Read the model definition and answer for the solid it produces. Units are mm, in the model's axes. Face numbers are marked on the shaded views. A direction names the side the tool comes from. Round coordinates to 2 decimals unless told otherwise and drop trailing zeros. Write each loop counter-clockwise with the first axis right and the second up, starting at its lowest first coordinate (ties: lowest second). Pieces come first, ordered by that corner, then holes. Notation, with made-up numbers: (-36.5, 47) -> (-20.5, 47) arc R8 cw to (-20.5, 53) -> close; hole circle Ø7 at (59.5, -37). An arc over 180 degrees is marked (long way). Return JSON: item names as keys, results as strings. Group by question number.
(1) The mould has two halves that part along Y. Classify the marked faces 1, 2 and 3: released by +Y, released by -Y, zero draft, split by the parting line, or undercut.
(2) A cutting plane is placed at B-B on y = 57. Give the vertices of the cut face in (x, z), then the cut area to 3 significant figures.
(3) A cutting plane is placed at D-D on x = 68.5. Give the vertices of the cut face in (y, z), then the cut area to 3 significant figures.
(4) A cutting plane is placed at A-A on x = 25. Give the vertices of the cut face in (y, z).
(5) A cutting plane is placed at C-C on z = -23. Give the vertices of the cut face in (x, y).
(6) Given pin 1 (6 mm diameter, centred on x = 26.5, y = 55.5, fed in from +Z); pin 2 (9.5 mm diameter, centred on x = 109, y = 57, fed in from -Z); pin 3 (1.8 mm diameter, centred on y = 2, z = -13, fed in from -X); pin 4 (1.8 mm diameter, centred on y = 1.5, z = -13, fed in from +X), each flat-ended and moving along its own axis, determine where each tip first touches the part or whether it passes through.
(7) Straight lines are drawn through the part: line 1 (Y direction, x = 25, z = 1.9); line 2 (Y direction, x = 76.5, z = -14); line 3 (Z direction, x = 98, y = 78.5). For each, find the intervals that lie inside material, in ascending order.
(8) For the marked faces 4 and 5, determine the directions among +Z, -Z, +X, -X, +Y, -Y from which every point of the face is accessible in a straight line to the end or side of a thin tool.
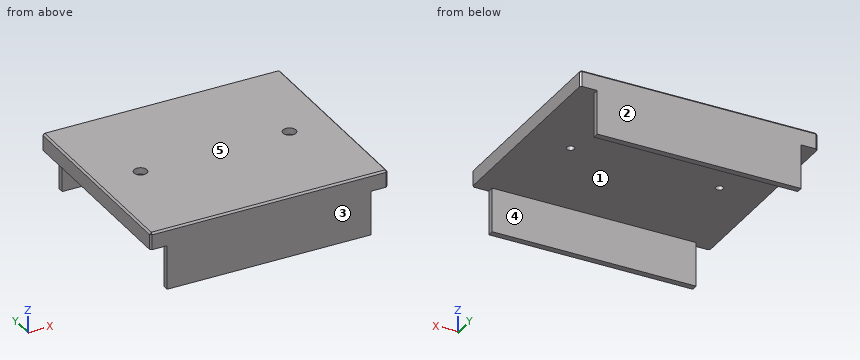
```python
from build123d import *

# Parameters (mm, degrees)
SKETCH1_W           = 134
SKETCH1_H           = 114
BOSS_EXTRUDE1_DEPTH = 9.5
SKETCH2_W           = 115
SKETCH2_H           = 3.5
BOSS_EXTRUDE2_DEPTH = 25
SKETCH3_R           = 2.15
CUT_EXTRUDE1_DEPTH  = 180.282598152
SKETCH4_R           = 3.65
CUT_EXTRUDE2_DEPTH  = 3.6
CHAMFER1_SIZE       = 1


with BuildPart() as part:
    # Sketch1 → Boss-Extrude1 (new body)
    with BuildSketch(Plane.XY):
        with Locations((67, 57)):
            Rectangle(SKETCH1_W, SKETCH1_H)
    extrude(amount=BOSS_EXTRUDE1_DEPTH)

    # Sketch2 → Boss-Extrude2 (add)
    with BuildSketch(Plane(origin=(0, 0, 0), x_dir=(-1, 0, 0), z_dir=(0, 0, -1))):
        Polygon((-67, 114), (-124.5, 114), (-124.5, 110.5), (-9.5, 110.5), (-9.5, 114), align=None)
        with Locations((-67, 1.75)):
            Rectangle(SKETCH2_W, SKETCH2_H)
    extrude(amount=BOSS_EXTRUDE2_DEPTH)

    # Sketch3 → Cut-Extrude1 (cut, through all)
    with BuildSketch(Plane.XY.offset(9.5)):
        with Locations((25, 57)):
            Circle(SKETCH3_R)
        with Locations((109, 57)):
            Circle(SKETCH3_R)
    extrude(amount=-CUT_EXTRUDE1_DEPTH, mode=Mode.SUBTRACT)

    # Sketch4 → Cut-Extrude2 (cut)
    with BuildSketch(Plane.XY.offset(9.5)):
        with Locations((25, 57)):
            Circle(SKETCH4_R)
        with Locations((109, 57)):
            Circle(SKETCH4_R)
    extrude(amount=-CUT_EXTRUDE2_DEPTH, mode=Mode.SUBTRACT)

    # Chamfer1
    chamfer1_edges = [part.edges().sort_by_distance(p)[0] for p in [
        (134, 57, 9.5),
        (67, 114, 9.5),
        (0, 57, 9.5),
        (67, 0, 9.5),
        (0, 114, 4.75),
        (134, 114, 4.75),
        (134, 0, 4.75),
        (0, 0, 4.75),
    ]]
    chamfer(chamfer1_edges, length=CHAMFER1_SIZE)


solid = part.part
```
Checks:
{
 "1": {"face 1": "undercut", "face 2": "released by +Y", "face 3": "released by -Y"},
 "2": {"outline": "(0, 0) -> (22.85, 0) -> (22.85, 5.9) -> (21.35, 5.9) -> (21.35, 9.5) -> (1, 9.5) -> (0, 8.5) -> close; (27.15, 0) -> (106.85, 0) -> (106.85, 5.9) -> (105.35, 5.9) -> (105.35, 9.5) -> (28.65, 9.5) -> (28.65, 5.9) -> (27.15, 5.9) -> close; (111.15, 0) -> (134, 0) -> (134, 8.5) -> (133, 9.5) -> (112.65, 9.5) -> (112.65, 5.9) -> (111.15, 5.9) -> close", "area": "1,170 mm^2"},
 "3": {"outline": "(0, -25) -> (3.5, -25) -> (3.5, 0) -> (110.5, 0) -> (110.5, -25) -> (114, -25) -> (114, 8.5) -> (113, 9.5) -> (1, 9.5) -> (0, 8.5) -> close", "area": "1,260 mm^2"},
 "4": {"outline": "(0, -25) -> (3.5, -25) -> (3.5, 0) -> (54.85, 0) -> (54.85, 5.9) -> (53.35, 5.9) -> (53.35, 9.5) -> (1, 9.5) -> (0, 8.5) -> close; (59.15, 0) -> (110.5, 0) -> (110.5, -25) -> (114, -25) -> (114, 8.5) -> (113, 9.5) -> (60.65, 9.5) -> (60.65, 5.9) -> (59.15, 5.9) -> close"},
 "5": {"outline": "(9.5, 0) -> (124.5, 0) -> (124.5, 3.5) -> (9.5, 3.5) -> close; (9.5, 110.5) -> (124.5, 110.5) -> (124.5, 114) -> (9.5, 114) -> close"},
 "6": {"pin 1": "stops at z = 9.5", "pin 2": "stops at z = 0", "pin 3": "stops at x = 9.5", "pin 4": "stops at x = 124.5"},
 "7": {"line 1": "y = 0 to 54.85, 59.15 to 114", "line 2": "y = 0 to 3.5, 110.5 to 114", "line 3": "z = 0 to 9.5"},
 "8": {"face 4": "-Z, +X, -X", "face 5": "+Z, +X, -X, +Y, -Y"}
}
